The model under review builds one solid part; all positions refer to its coordinate system, in mm. A direction names the side the tool comes from. Coordinates: 2 decimals unless noted, no trailing zeros. Write each loop counter-clockwise with the first axis right and the second up, starting at its lowest first coordinate (ties: lowest second). Pieces come first, ordered by that corner, then holes. Notation, with made-up numbers: (64, -15.75) - (102, -15.75) arc R12 ccw to (102, -5.75) - close; hole circle Ø1 at (26.5, 19.25). An arc over 180 degrees is marked (long way). Put each result on its own line as item: value. Start each with the question number.
Item 1: Machinability: for faces 5 (the face through (48, 0, 76)), 6 (the face through (73.273, -6.439, 56.184)), which of the approach directions +Z, -Z, +X, -X, +Y, -Y give a long, thin tool a straight path to every point of the face, cutting with its end or side? Answer none if there is none.
Item 2: Consider section A-A on x = 0. Give the boundary of the cut face in (y, z).
Item 3: Consider section D-D on y = -78. Give the boundary of the cut face in (x, z), then the cut area to 3 significant figures.
Item 4: Consider section B-B on z = 0. Give the boundary of the cut face in (x, y), then the cut area to 3 significant figures.
Item 5: Mouldability with a two-part tool opening along X and no side actions: class faces 1 (the face through (47.3, -47.3, -36.3)), 2 (the face through (13.416, -67.648, -60.417)), 3 (the face through (28, -12.7, 69)), 4 (the face through (16.075, 18.403, -72.39)) as pulls with the +X half, pulls with the -X half, needs draft (parallel to the pull), parting line crosses it, or undercut.
Item 6: Consider section C-C on y = -26. Give the boundary of the cut face in (x, z), then the cut area to 3 significant figures.
Item 7: To check wall thickness, follow L1, parallel to X at y = -65, z = 32.5; L2, parallel to Y at x = -42, z = -81; L3, parallel to Z at x = -55.5, y = -7.5. State the ranges of each line that lie inside material, in increasing order. Write a range as [from, to].
Item 8: For pin 1 (12 mm diameter, centred on x = -49, y = -56, fed in from +Z); pin 2 (6 mm diameter, centred on x = 21.5, y = -15, fed in from +Z); pin 3 (5 mm diameter, centred on x = -27.5, y = -80.5, fed in from -Z), all flat-tipped, find the tip position at first contact; note any pin that passes through.
Autodesk Inventor part; units mm, degrees
ref_plane "YZ Plane" through (0, 0, 0) normal (1, 0, 0) x (0, 1, 0)
ref_plane "XZ Plane" through (0, 0, 0) normal (0, 1, 0) x (-1, 0, 0)
ref_plane "XY Plane" through (0, 0, 0) normal (0, 0, 1) x (1, 0, 0)
sketch "Sketch1" plane through (0, 0, 0) normal (0, 0, 1) x (1, 0, 0)
  line L0 (0, 25.4) -> (-28.702, 25.4) construction
  line L1 (0, 25.4) -> (-95.25, 25.4) construction
  line L2 (-95.25, 25.4) -> (-89.1588, 25.4) construction
  line L3 (-89.1588, 25.4) -> (-85.693, 23.7839) construction
  line L4 (-89.1588, 25.4) -> (-89.1588, 21.1626) construction
  line L5 (-89.1588, 0) -> (-92.3338, 0)
  line L6 (-28.702, 59.6457) -> (-28.702, -91.9304) construction
  arc A0 (-28.9184, -8.4804) -> (-32.3684, -1.0818) centre (-35.052, -6.8369) ccw
  line L7 (-89.1588, 25.4) -> (-89.1588, 0)
  line L8 (-89.1588, 25.4) -> (-32.3684, -1.0818)
  line L9 (-28.9184, -8.4804) -> (-28.9392, -8.5583)
  line L10 (0, -319.0244) -> (0, 122.7573)
  line L11 (-73.152, 17.9359) -> (-28.702, 17.9359) construction
  line L12 (-89.1588, 0) -> (-92.3338, 0)
  line L13 (11.4547, -6.8369) -> (-136.2084, -6.8369) construction
  line L14 (-57.2892, -89.8271) -> (-74.8171, -155.2422)
  line L15 (-92.3338, -12.7) -> (-73.2838, -12.7)
  line L16 (-73.2838, -12.7) -> (-54.421, -103.6575)
  line L17 (-74.8171, -155.2422) -> (-68.2431, -155.2422)
  line L18 (-92.3338, -25.4) -> (-79.6338, -25.4)
  line L19 (-79.6338, -25.4) -> (-79.6338, -57.15)
  line L20 (-79.6338, -57.15) -> (-72.991, -88.4936)
  line L21 (-92.3338, 0) -> (-92.3338, -25.4)
  line L22 (-86.3902, -25.4) -> (-86.3902, -31.3436)
  line L23 (-86.3902, -31.3436) -> (-92.3338, -31.3436)
  line L24 (-92.3338, -31.3436) -> (-92.3338, -56.7436)
  line L25 (-92.3338, -56.7436) -> (-79.6338, -56.7436)
  line L26 (-73.152, 17.9359) -> (-32.3684, -1.0818)
  line L27 (-73.152, 17.9359) -> (-50.7653, -90.0141)
  line L28 (-50.7653, -90.0141) -> (-28.9184, -8.4804)
  line L29 (-52.4654, -96.3589) -> (-28.9184, -8.4804)
  line L30 (-86.36, -222.8555) -> (-28.9184, -8.4804)
  line L31 (-72.991, -88.4936) -> (-89.535, -222.8555)
  line L32 (-89.535, -222.8555) -> (-86.36, -222.8555)
  line L33 (-54.421, -103.6575) -> (-50.7653, -90.0141)
  line L34 (-73.152, 17.9359) -> (-89.1588, 25.4)
  line L35 (-89.1588, 0) -> (-89.1588, 25.4)
  line L36 (-89.1588, 0) -> (-92.3338, 0)
  line L37 (-92.3338, -12.7) -> (-73.2838, -12.7)
  line L38 (-73.2838, -12.7) -> (-54.421, -103.6575)
  line L39 (-92.3338, -12.7) -> (-92.3338, 0)
  point P0 (0, 0)
  point P1 (-95.25, -255.9127)
  point P2 (-88.7095, 22.4389)
  dimension "d0" = 28.702
  dimension "d3" = 25
  dimension "d5" = 25.4
  dimension "d6" = 25.4
  dimension "d8" = 12.7
  dimension "d34" = 15
  dimension "d37" = 44.45
  dimension "d46" = 19.05
  dimension "d47" = 12.7
  dimension "d55" = 12.7
  dimension "d56" = 31.75
  dimension "d58" = 0.25
  dimension "d60" = 12.7
  dimension "d61" = 25.4
  dimension "d62" = 5.9436
  dimension "d63" = 5.9436
  dimension "d64" = 3.175
  dimension "d68" = 107.95
  dimension "d69" = 6.35
  dimension "d70" = 6.35
  dimension "d71" = 3.175
  dimension "d73" = 86.36
  dimension "d74" = 31.75
  dimension "d75" = 6.3448
revolve "Revolution3" add sketch "Sketch1" angle 360 about axis through (0, -10, 0) along (0, 1, 0) contours L7 L8 L27 L29 L30 L16 L15 L21 L5
properties part number "phenolic_top" material "Phenolic Resin"
Report:
1. face 5: +Y
1. face 6: +Y, -Y
2. outline: (-103.66, -54.42) - (-12.7, -73.28) - (-12.7, -92.33) - (0, -92.33) - (0, -89.16) - (25.4, -89.16) - (17.94, -73.15) - (-90.01, -50.77) - (-96.36, -52.47) - close; (-103.66, 54.42) - (-96.36, 52.47) - (-90.01, 50.77) - (17.94, 73.15) - (25.4, 89.16) - (0, 89.16) - (0, 92.33) - (-12.7, 92.33) - (-12.7, 73.28) - close
3. outline: circle Ø119.48 at (0, 0); hole circle Ø106.51 at (0, 0)
3. area: 2,300 mm²
4. outline: (-92.33, -12.7) - (-73.28, -12.7) - (-54.42, -103.66) - (-52.47, -96.36) - (-50.77, -90.01) - (-73.15, 17.94) - (-89.16, 25.4) - (-89.16, 0) - (-92.33, 0) - close; (50.77, -90.01) - (52.47, -96.36) - (54.42, -103.66) - (73.28, -12.7) - (92.33, -12.7) - (92.33, 0) - (89.16, 0) - (89.16, 25.4) - (73.15, 17.94) - close
4. area: 2,470 mm²
5. face 1: undercut
5. face 2: parting line crosses it
5. face 3: needs draft
5. face 4: undercut
6. outline: circle Ø141.05 at (0, 0); hole circle Ø128.08 at (0, 0)
6. area: 2,740 mm²
7. L1: [-53.31, -45.55], [45.55, 53.31]
7. L2: [-12.7, 0]
7. L3: [-73.79, -39.08], [39.08, 73.79]
8. pin 1: z = 48.07
8. pin 2: z = 90.24
8. pin 3: z = -53.82
